Read the model definition and answer for the solid it produces. Units are mm, in the model's axes. A direction names the side the tool comes from. Coordinates: 2 decimals unless noted, no trailing zeros. Loops run counter-clockwise (first coordinate to the right, second up) from the corner with the lowest first, then second, coordinate; pieces in that order, holes last.
Q1. Flat-ended cylindrical pins translate along their axes: P1, Ø4, axis at x = -17.58, z = -57, coming from the -Y side; P2, Ø2.5, axis at y = 2, z = -111, coming from the +X side. Find the tip coordinate at first contact, or state that the pin passes through.
Q2. Section A-A (z = -86.5) is taken. Give the vertices of the cut face in (x, y).
Q3. The mould has two halves that part along Z. Classify faces 3 (the face through (45, 0, -23)), 4 (the face through (42, 2, -126.088)), 5 (the face through (-18.57, 2.35, -55.09)): pulls with the +Z half, pulls with the -Z half, needs draft (parallel to the pull), parting line crosses it, or undercut.
Q4. Straight lines are drawn through the part: line 1 (X direction, y = 0.2, z = -55.5); line 2 (X direction, y = 3.7, z = -103.5). For each, find the intervals that lie inside material, in ascending order.
Q5. Which of the six approach directions +Z, -Z, +X, -X, +Y, -Y give full straight-line access (tool end or side, diameter ignored) to faces 1 (the face through (113.737, 2, 6)), 2 (the face through (108.962, 2, -99))?
from build123d import *

# Parameters (mm, degrees)
SKETCH1_W             = 136.525
SKETCH1_H             = 209.55
BOSS_EXTRUDE1_DEPTH   = 4.7625
SKETCH2_W             = 4.7752
SKETCH2_H             = 53.34
CUT_EXTRUDE1_DEPTH    = 170.873266436
F_8_CLEARANCE_HOLE1_D = 4.3053


with BuildPart() as part:
    # Sketch1 → Boss-Extrude1 (new body)
    with BuildSketch(Plane(origin=(0, 0, 0), x_dir=(1, 0, 0), z_dir=(0, 1, 0))):
        with Locations((45.474550145, 21.312781595)):
            Rectangle(SKETCH1_W, SKETCH1_H)
    extrude(amount=BOSS_EXTRUDE1_DEPTH)

    # Sketch2 → Cut-Extrude1 (cut, through all)
    with BuildSketch(Plane(origin=(0, 4.7625, 0), x_dir=(1, 0, 0), z_dir=(0, 1, 0))):
        with Locations((111.349450145, 99.417781595)):
            Rectangle(SKETCH2_W, SKETCH2_H)
    extrude(amount=-CUT_EXTRUDE1_DEPTH, mode=Mode.SUBTRACT)

    # #8 Clearance Hole1 (through all)
    with Locations(Plane(origin=(0, 4.7625, 0), x_dir=(1, 0, 0), z_dir=(0, 1, 0))):
        with Locations((81.161550145, -72.540218405), (9.787550145, -72.540218405), (-17.580949855, 56.999781595), (108.530050145, 56.999781595)):
            Hole(F_8_CLEARANCE_HOLE1_D / 2)


solid = part.part
Numbers:
1. P1: passes through
1. P2: stops at x = 108.96
2. outline: (-22.79, 0) - (108.96, 0) - (108.96, 4.76) - (-22.79, 4.76) - close
3. face 3: needs draft
3. face 4: pulls with the -Z half
3. face 5: undercut
4. line 1: x = -22.79 to -19.13, -16.04 to 106.99, 110.07 to 113.74
4. line 2: x = -22.79 to 108.96
5. face 1: +Z, -Z, +X, +Y, -Y
5. face 2: -Z, +X, +Y, -Y
